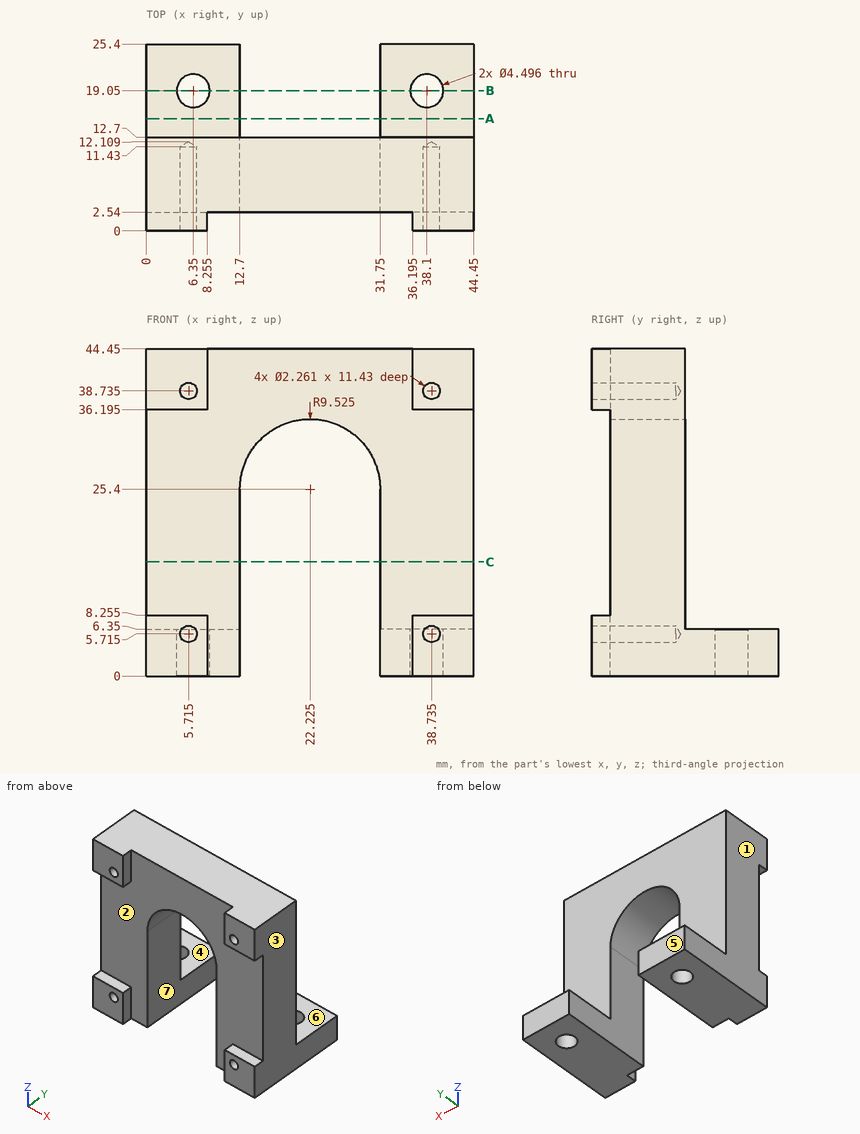
Drawing for the job (mm, zero at the part's lowest x, y, z). A direction names the side the tool comes from. Round coordinates to 2 decimals unless told otherwise and drop trailing zeros. Order: outer loops, then holes, each group sorted by start corner. A loop starts at its lowest first (then second) coordinate and runs counter-clockwise, first axis right, second up. Notation, with made-up numbers: (0, 4) -> (14, 4) arc R30 cw to (14, 31) -> close; hole circle Ø9 at (27.25, -3). An arc over 180 degrees is marked (long way). Write item = value, one per line. Start each with the question number.
(1) Pull direction X, two halves, no side cores. Call the marked faces 1, 2, 3 and 4: released by +X, released by -X, zero draft, split by the parting line, or undercut.
(2) Which spindle directions (+Z, -Z, +X, -X, +Y, -Y) get a long thin tool onto all of the face, cutting with end or side? Do the marked faces 5, 6 and 7. Say none if no direction does.
(3) Cut at A-A, the plane y = 15.25. List the corners of the cut face in (x, z), then the cut area to 3 significant figures.
(4) Probe line 1 (Y direction, x = 6.35, z = 4.5); line 2 (X direction, y = 12.5, z = 17); line 3 (Y direction, x = 32, z = 6.5). List the from-to ranges inside material, lowest first. Write a range as [from, to].
(5) Pin check, flat tips, straight feed: P1, Ø3, axis at x = 34.5, z = 6.5, coming from the -Y side; P2, Ø1.4, axis at x = 38.735, z = 38.735, coming from the -Y side; P3, Ø1.5, axis at x = 15, y = 5.5, coming from the -Z side. Stop position of each tip, or through.
(6) Cut at C-C, the plane z = 15.5. List the corners of the cut face in (x, y), then the cut area to 3 significant figures.
(7) Cut at B-B, the plane y = 19.05. List the corners of the cut face in (x, z).
Model answer:
q1.face_1 = released by -X
q1.face_2 = undercut
q1.face_3 = released by +X
q1.face_4 = zero draft
q2.face_5 = +Z, -Z, +X, -X, +Y
q2.face_6 = +Z, +X, -X, +Y
q2.face_7 = -Z, +Y, -Y
q3.outline = (0, 0) -> (12.7, 0) -> (12.7, 6.35) -> (0, 6.35) -> close; (31.75, 0) -> (44.45, 0) -> (44.45, 6.35) -> (31.75, 6.35) -> close
q3.area = 161 mm2
q4.line_1 = [0, 16.8], [21.3, 25.4]
q4.line_2 = [0, 12.7], [31.75, 44.45]
q4.line_3 = [2.54, 12.7]
q5.P1 = 2.54
q5.P2 = 11.69
q5.P3 = 30.61
q6.outline = (0, 2.54) -> (12.7, 2.54) -> (12.7, 12.7) -> (0, 12.7) -> close; (31.75, 2.54) -> (44.45, 2.54) -> (44.45, 12.7) -> (31.75, 12.7) -> close
q6.area = 258 mm2
q7.outline = (0, 0) -> (4.1, 0) -> (4.1, 6.35) -> (0, 6.35) -> close; (8.6, 0) -> (12.7, 0) -> (12.7, 6.35) -> (8.6, 6.35) -> close; (31.75, 0) -> (35.85, 0) -> (35.85, 6.35) -> (31.75, 6.35) -> close; (40.35, 0) -> (44.45, 0) -> (44.45, 6.35) -> (40.35, 6.35) -> close
